```python
from build123d import *

# Parameters (mm, degrees)
SKETCH1_R                 = 28
BOSS_EXTRUDE1_DEPTH       = 14
SKETCH2_R                 = 15
CUT_EXTRUDE1_DEPTH        = 8
CUT_EXTRUDE2_DEPTH        = 16
M5X0_8_TAPPED_HOLE1_D     = 4.2
M5X0_8_TAPPED_HOLE1_DEPTH = 8
M5X0_8_TAPPED_HOLE1_TIP   = 1.2618073


with BuildPart() as part:
    # Sketch1 → Boss-Extrude1 (new body)
    with BuildSketch(Plane.YZ):
        with Locations(Location((0, 0, 0), (0, 0, 270))):
            Circle(SKETCH1_R)
    extrude(amount=BOSS_EXTRUDE1_DEPTH)

    # Sketch2 → Cut-Extrude1 (cut)
    with BuildSketch(Plane.YZ.offset(14)):
        with Locations(Location((0, 0, 0), (0, 0, 270))):
            Circle(SKETCH2_R)
    extrude(amount=-CUT_EXTRUDE1_DEPTH, mode=Mode.SUBTRACT)

    # Sketch3 → Cut-Extrude2 (cut)
    with BuildSketch(Plane(origin=(0, 0, 0), x_dir=(0, -1, 0), z_dir=(-1, 0, 0))):
        with BuildLine():
            Line((-2, 7.5), (2, 7.5))
            Line((2, 7.5), (2, 5.656854249))
            ThreePointArc((2, 5.656854249), (0, -6), (-2, 5.656854249))
            Line((-2, 5.656854249), (-2, 7.5))
        make_face()
    extrude(amount=-CUT_EXTRUDE2_DEPTH, mode=Mode.SUBTRACT)

    # M5x0.8 Tapped Hole1
    with Locations(Plane(origin=(14, -20.4477151, 6.643865379), x_dir=(0, 0, 1), z_dir=(1, 0, 0))):
        with Locations((0, 0), (14.856134621, -20.4477151), (-24.037730758, -7.810332176), (-24.037730758, -33.085098024), (0, -40.8954302)):
            Hole(M5X0_8_TAPPED_HOLE1_D / 2, depth=M5X0_8_TAPPED_HOLE1_DEPTH)
            with Locations((0, 0, -(M5X0_8_TAPPED_HOLE1_DEPTH + M5X0_8_TAPPED_HOLE1_TIP / 2))):  # 118° drill point
                Cone(0, M5X0_8_TAPPED_HOLE1_D / 2, M5X0_8_TAPPED_HOLE1_TIP, mode=Mode.SUBTRACT)


solid = part.part
```
Verification items for the finished model (mm, model axes). A direction names the side the tool comes from. Round coordinates to 2 decimals unless told otherwise and drop trailing zeros. Write each loop counter-clockwise with the first axis right and the second up, starting at its lowest first coordinate (ties: lowest second). Pieces come first, ordered by that corner, then holes. Notation, with made-up numbers: (82.25, 42.25) -> (141.25, 42.25) arc R20 cw to (141.25, 68.25) -> close; hole circle Ø9 at (14, 37.25). An arc over 180 degrees is marked (long way). Write each question's results on one line, items separated by ' | '.
Q1. Draft check along Y on faces 4 (the face through (3, 0, -6)), 5 (the face through (14, -12, -12)), 6 (the face through (6.902, -27.334, 6.07)). Enter one of: released by +Y, released by -Y, zero draft, split by the parting line, or undercut.
Derived:
face 4: undercut | face 5: zero draft | face 6: split by the parting line
Q2. Sectioned sample at D-D, the plane x = 1.75. Record the boundary of the cut face in (y, z).
Derived:
outline: circle Ø56 at (0, 0); hole (-2, 5.66) arc R6 ccw (long way) to (2, 5.66) -> (2, 7.5) -> (-2, 7.5) -> close
Q3. Sectioned sample at C-C, the plane y = 9. Record the boundary of the cut face in (x, z), and give its area (3 significant figures).
Derived:
outline: (0, -26.51) -> (14, -26.51) -> (14, -12) -> (6, -12) -> (6, 12) -> (14, 12) -> (14, 26.51) -> (0, 26.51) -> close | area: 550 mm²
Q4. Thickness scan on probe 1 along Y at (x, z) = (10.5, 0); probe 2 along Z at (x, y) = (6.25, 13.5); probe 3 along X at (y, z) = (12, 7). Record the ranges inside material, lowest first.
Derived:
probe 1: y = -28 to -15, 15 to 28 | probe 2: z = -24.53 to -19.31, -15.48 to -6.54, 6.54 to 24.53 | probe 3: x = 0 to 6
Q5. Sectioned sample at B-B, the plane x = 7.75. Record the boundary of the cut face in (y, z).
Derived:
outline: circle Ø56 at (0, 0); hole circle Ø4.2 at (-20.45, 6.64); hole circle Ø30 at (0, 0); hole circle Ø4.2 at (-12.64, -17.39); hole circle Ø4.2 at (0, 21.5); hole circle Ø4.2 at (12.64, -17.39); hole circle Ø4.2 at (20.45, 6.64)
Q6. Sectioned sample at A-A, the plane z = 0. Record the boundary of the cut face in (x, y), and give its area (3 significant figures).
Derived:
outline: (0, -28) -> (14, -28) -> (14, -15) -> (6, -15) -> (6, -6) -> (0, -6) -> close; (0, 6) -> (6, 6) -> (6, 15) -> (14, 15) -> (14, 28) -> (0, 28) -> close | area: 472 mm²
Q7. Access from +Z, -Z, +X, -X, +Y, -Y to the whole of each face (thin tool, end or side, straight path). Record for faces 1 (the face through (3, -2, 7)), 2 (the face through (9.94, 18.68, 5.51)), 3 (the face through (0, 7, 0)).
Derived:
face 1: +X, -X | face 2: +X | face 3: +Z, -Z, -X, +Y, -Y
Q8. Go/stop test with flat-tipped pins: pin 1 Ø3.5 at (y, z) = (20.45, 6.64) entering from +X; pin 2 Ø1 at (x, y) = (4.5, -12) entering from +Z; pin 3 Ø1.5 at (x, z) = (3, 7) entering from +Y. Record where each tip stops, or that it passes through.
Derived:
pin 1: stops at x = 5.79 | pin 2: stops at z = 25.53 | pin 3: stops at y = 27.29
